The figure shows three views and two pictorial views of one solid part (mm, origin at its lowest corner). Answer the questions. A direction names the side the tool comes from. Coordinates: 2 decimals unless noted, no trailing zeros. Loops run counter-clockwise (first coordinate to the right, second up) from the corner with the lowest first, then second, coordinate; pieces in that order, holes last. Notation, with made-up numbers: (8, -25.75) -> (55, -25.75) arc R33 cw to (55, 5.25) -> close; hole circle Ø10 at (25, 73.25). An arc over 180 degrees is marked (long way). Answer in a Markdown table with one row per item.
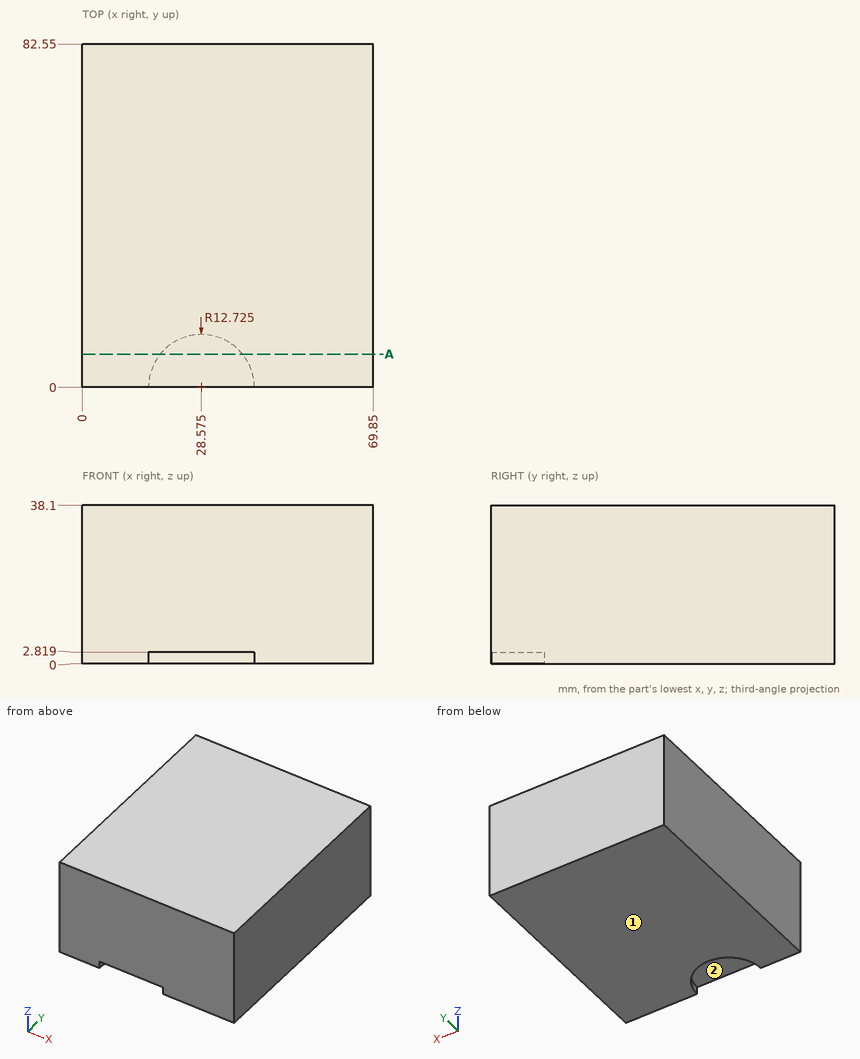
Item 1: A tool of negligible diameter and unlimited length cuts with its end or side. For the marked faces 1 and 2, from which of +Z, -Z, +X, -X, +Y, -Y can it reach the whole face along a straight path? Write none if from no direction.
Findings below:
| item | result |
|---|---|
| face 1 | -Z, +X, -X, +Y, -Y |
| face 2 | -Z, -Y |
Item 2: A flat-ended cylindrical pin translates along its axis: pin 1 Ø14 at (x, y) = (30.5, 4) entering from -Z. Find the tip coordinate at first contact, or state that the pin passes through.
Findings below:
| item | result |
|---|---|
| pin 1 | stops at z = 2.82 |
Item 3: A cutting plane is placed at A-A, the plane y = 8. Determine the outline of the cut face in (x, z), plus the area to 3 significant figures.
Findings below:
| item | result |
|---|---|
| outline | (0, 0) -> (18.68, 0) -> (18.68, 2.82) -> (38.47, 2.82) -> (38.47, 0) -> (69.85, 0) -> (69.85, 38.1) -> (0, 38.1) -> close |
| area | 2,610 mm2 |
